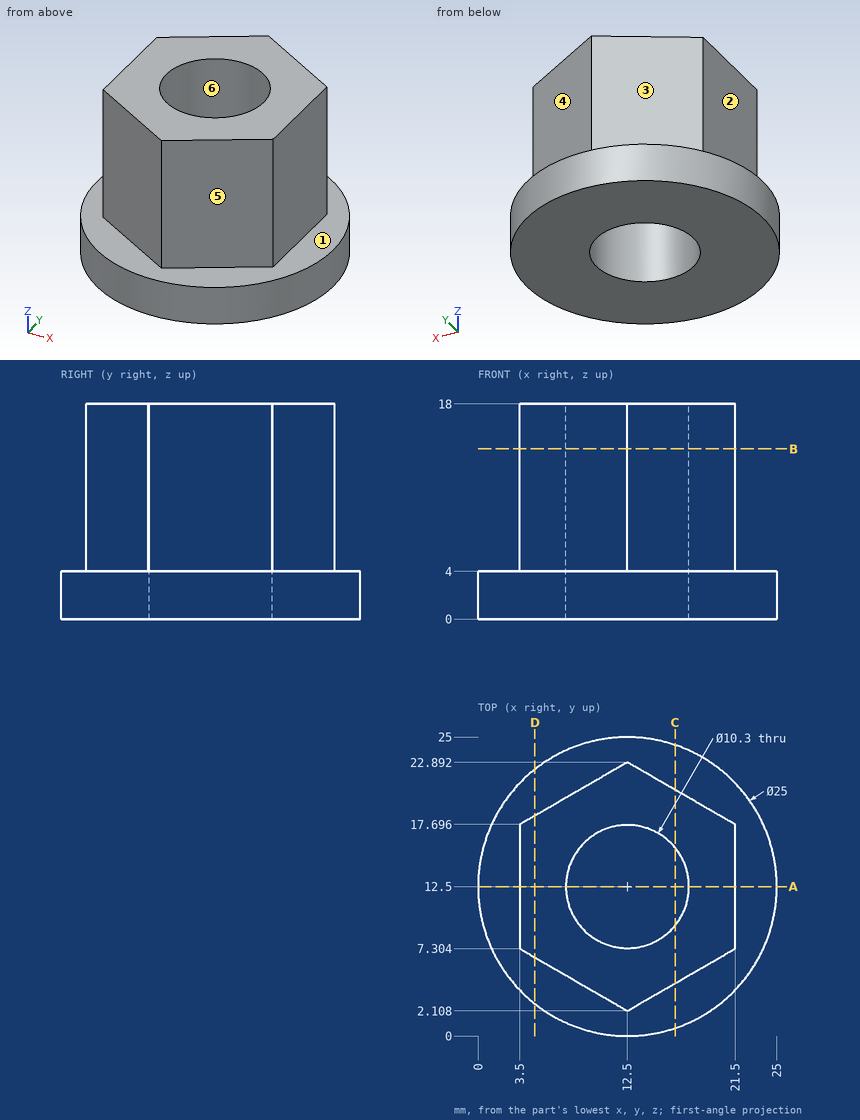
For this review, use the dimensioned drawing (mm, ordinates from the lowest corner) and the shaded views. A direction names the side the tool comes from. Coordinates: 2 decimals unless noted, no trailing zeros. Write each loop counter-clockwise with the first axis right and the second up, starting at its lowest first coordinate (ties: lowest second). Pieces come first, ordered by that corner, then holes. Notation, with made-up numbers: (34, 6.5) -> (90, 6.5) arc R30 ccw to (90, 33.5) -> close; hole circle Ø3 at (69.25, 71). An arc over 180 degrees is marked (long way). Write each question's results on one line, items separated by ' | '. Start each with the question number.
(1) Take a section at B-B on z = 14.25. Write out the cut boundary in (x, y), and give its area (3 significant figures).
(2) Take a section at D-D on x = 4.75. Write out the cut boundary in (y, z), and give its area (3 significant figures).
(3) Tool access review of the marked faces 1, 2 and 3: name each direction out of +Z, -Z, +X, -X, +Y, -Y from which nothing blocks a thin tool from reaching the whole face with its end or side.
(4) Take a section at C-C on x = 16.5. Write out the cut boundary in (y, z).
(5) Take a section at A-A on y = 12.5. Write out the cut boundary in (x, z), and give its area (3 significant figures).
(6) Clearance check with flat-ended pins moving along their axes: P1, Ø5, axis at y = 4.5, z = 2.5, coming from the -X side (1 decimal); P2, Ø5, axis at y = 12, z = 13.5, coming from the -X side; P3, Ø5, axis at y = 3, z = 12, coming from the -X side (1 decimal); P4, Ø3, axis at x = 20, y = 7.5, coming from the -Z side. State where each tip first meets the part, or that it passes through.
(7) For line 1 along X through (y, z) = (12.25, 12.25); line 2 along Z through (x, y) = (18, 22.75); line 3 along Y through (x, z) = (12.25, 15.5) (1 decimal), list the stretches that pass through material, from the lowest coordinate up. Write a range as from..to.
(8) The part is to be moulded in two halves that separate along Y. For the marked faces 4, 5 and 6, say which applies: pulls with the +Y half, pulls with the -Y half, needs draft (parallel to the pull), parting line crosses it, or undercut.
Results found:
1) outline: (3.5, 7.3) -> (12.5, 2.11) -> (21.5, 7.3) -> (21.5, 17.7) -> (12.5, 22.89) -> (3.5, 17.7) -> close; hole circle Ø10.3 at (12.5, 12.5) | area: 197 mm2
2) outline: (2.69, 0) -> (22.31, 0) -> (22.31, 4) -> (18.42, 4) -> (18.42, 18) -> (6.58, 18) -> (6.58, 4) -> (2.69, 4) -> close | area: 244 mm2
3) face 1: +Z | face 2: +Z, -X, +Y, -Y | face 3: +Z, -X, +Y
4) outline: (0.66, 0) -> (9.26, 0) -> (9.26, 18) -> (4.42, 18) -> (4.42, 4) -> (0.66, 4) -> close; (15.74, 0) -> (24.34, 0) -> (24.34, 4) -> (20.58, 4) -> (20.58, 18) -> (15.74, 18) -> close
5) outline: (0, 0) -> (7.35, 0) -> (7.35, 18) -> (3.5, 18) -> (3.5, 4) -> (0, 4) -> close; (17.65, 0) -> (25, 0) -> (25, 4) -> (21.5, 4) -> (21.5, 18) -> (17.65, 18) -> close | area: 167 mm2
6) P1: stops at x = 1.3 | P2: stops at x = 3.5 | P3: stops at x = 6.6 | P4: stops at z = 0
7) line 1: x = 3.5..7.36, 17.64..21.5 | line 2: z = 0..4 | line 3: y = 2.3..7.4, 17.6..22.7
8) face 4: pulls with the +Y half | face 5: pulls with the -Y half | face 6: undercut
